Part model, mm, in its own coordinate system. A direction names the side the tool comes from. Give positions to 0.01 mm unless a question says otherwise; leave off trailing zeros. Write each loop counter-clockwise with the first axis right and the second up, starting at its lowest first coordinate (ties: lowest second). Pieces come first, ordered by that corner, then holes. Notation, with made-up numbers: M 30,55.25 L 47,55.25 A22 cw 47,70.25 Z; hole C 29.5,-10.75 d10. An arc over 180 degrees is marked long. Use a Markdown table: item, result. Add a question column.
from build123d import *

# Parameters (mm, degrees)
SKETCH1_W           = 38
SKETCH1_H           = 15
SKETCH1_R           = 4.875
BOSS_EXTRUDE1_DEPTH = 1.5
SKETCH1_3_R         = 4.875
BOSS_EXTRUDE2_DEPTH = 10


with BuildPart() as part:
    # Sketch1 → Boss-Extrude1 (new body)
    # profile 1 of 2: a face of its own
    with BuildSketch(Plane(origin=(0, 0, 0), x_dir=(1, 0, 0), z_dir=(0, 1, 0))):
        Rectangle(SKETCH1_W, SKETCH1_H)
        with Locations((10.09, 0)):
            Circle(SKETCH1_R, mode=Mode.SUBTRACT)
    # profile 2 of 2: a face of its own
    with BuildSketch(Plane(origin=(0, 0, 0), x_dir=(1, 0, 0), z_dir=(0, 1, 0))):
        with Locations((10.09, 0)):
            Circle(SKETCH1_R)
    extrude(amount=-BOSS_EXTRUDE1_DEPTH)

    # Sketch1_3 → Boss-Extrude2 (add)
    with BuildSketch(Plane(origin=(0, 0, 0), x_dir=(1, 0, 0), z_dir=(0, 1, 0))):
        with Locations(Location((10.09, 0, 0), (0, 0, 270))):
            Circle(SKETCH1_3_R)
    extrude(amount=BOSS_EXTRUDE2_DEPTH)


solid = part.part
1. Cut at D-D (z = -5.25). Write the cut outline in (x, y), then the cut area to 3 significant figures.
2. Cut at C-C (y = 6.5). Write the cut outline in (x, z) (3 decimals), then the cut area to 3 significant figures.
3. Tool access for faces 1 (the flat face through (-19, -1, 0)), 2 (the cylindrical face through (14.924, 4.93, -0.635)): list every direction of +Z, -Z, +X, -X, +Y, -Y with a clear straight run to the whole face (end or side of a thin tool).
4. Cut at A-A (z = 0). Write the cut outline in (x, y) (3 decimals), then the cut area to 4 significant figures.
5. Drill centre lines: probe 1 along Y at (x, z) = (-10, 1); probe 2 along X at (y, z) = (4.75, 0) (3 decimals); probe 3 along Z at (x, y) = (10, 5.5). Where is each one in solid material? Low to high. Write a range as [from, to].
6. Flat gauge pins, fed straight in: pin 1 (8 mm diameter, centred on x = -10.5, z = -5, fed in from +Y); pin 2 (2 mm diameter, centred on y = 8, z = -1.5, fed in from +X); pin 3 (3 mm diameter, centred on x = 11.5, y = 8, fed in from -Z) (3 decimals). Where does each tip first touch, or does it go through?
7. Cut at B-B (x = 10.09). Write the cut outline in (y, z) (3 decimals), then the cut area to 3 significant figures.
A:
| question | item | result |
|---|---|---|
| 1 | outline | M -19,-1.5 L 19,-1.5 L 19,0 L -19,0 Z |
| 1 | area | 57.0 mm² |
| 2 | outline | C 10.09,0 d9.75 |
| 2 | area | 74.7 mm² |
| 3 | face 1 | +Z, -Z, -X, +Y, -Y |
| 3 | face 2 | +Y |
| 4 | outline | M -19,-1.5 L 19,-1.5 L 19,0 L 14.965,0 L 14.965,10 L 5.215,10 L 5.215,0 L -19,0 Z |
| 4 | area | 154.5 mm² |
| 5 | probe 1 | y = [-1.5, 0] |
| 5 | probe 2 | x = [5.215, 14.965] |
| 5 | probe 3 | z = [-4.87, 4.87] |
| 6 | pin 1 | stops at y = 0 |
| 6 | pin 2 | stops at x = 14.94 |
| 6 | pin 3 | stops at z = -4.875 |
| 7 | outline | M -1.5,-7.5 L 0,-7.5 L 0,-4.875 L 10,-4.875 L 10,4.875 L 0,4.875 L 0,7.5 L -1.5,7.5 Z |
| 7 | area | 120 mm² |
